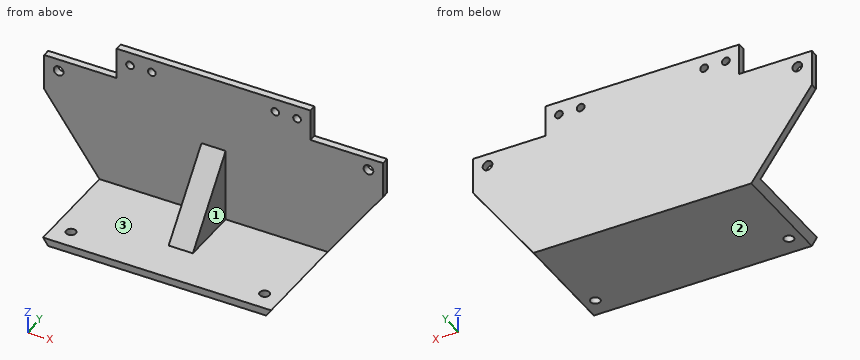
```python
from build123d import *

# Parameters (mm, degrees)
EXTRUDE_1_DEPTH     = 140
CUT_EXTRUDE_1_REACH = 152.354
SKETCH_2_R          = 2
CUT_EXTRUDE_2_REACH = 151.164
SKETCH_3_R          = 2
CUT_EXTRUDE_3_DEPTH = 150.164338902
RIB_2_REACH         = 79.661
SKETCH_9_WALL_W     = 196.169186172
SKETCH_9_WALL_H     = 10
SKETCH_10_W         = 80
SKETCH_10_H         = 3
EXTRUDE_2_DEPTH     = 13
SKETCH_11_R         = 1.6
CUT_EXTRUDE_4_DEPTH = 3


with BuildPart() as part:
    # 草图1 → 凸台-拉伸1 (new body)
    with BuildSketch(Plane(origin=(0, 0, 0), x_dir=(0, 0, -1), z_dir=(1, 0, 0))):
        Polygon((22, 19.5), (22, -22.5), (25, -22.5), (25, 22.5), (-25, 22.5), (-25, 19.5), align=None)
    extrude(amount=EXTRUDE_1_DEPTH)

    # 草图2 → 切除-拉伸1 (cut, up to next)
    with BuildSketch(Plane(origin=(0, 0, -25), x_dir=(-1, 0, 0), z_dir=(0, 0, -1)), mode=Mode.PRIVATE) as cut_extrude_1_sk1:
        with Locations((-110, -14.5)):
            Circle(SKETCH_2_R)
    cut_extrude_1_tool1 = extrude(cut_extrude_1_sk1.sketch, amount=-CUT_EXTRUDE_1_REACH, mode=Mode.PRIVATE) & part.part
    # 草图2 → 切除-拉伸1 (cut, up to next)
    with BuildSketch(Plane(origin=(0, 0, -25), x_dir=(-1, 0, 0), z_dir=(0, 0, -1)), mode=Mode.PRIVATE) as cut_extrude_1_sk2:
        with Locations((-30, -14.5)):
            Circle(SKETCH_2_R)
    cut_extrude_1_tool2 = extrude(cut_extrude_1_sk2.sketch, amount=-CUT_EXTRUDE_1_REACH, mode=Mode.PRIVATE) & part.part
    add(cut_extrude_1_tool1.solids().sort_by_distance((110, -14.5, -25))[0], mode=Mode.SUBTRACT)
    add(cut_extrude_1_tool2.solids().sort_by_distance((30, -14.5, -25))[0], mode=Mode.SUBTRACT)

    # 草图3 → 切除-拉伸2 (cut, up to next)
    with BuildSketch(Plane(origin=(0, 22.5, 0), x_dir=(1, 0, 0), z_dir=(0, 1, 0)), mode=Mode.PRIVATE) as cut_extrude_2_sk1:
        with Locations(Location((6, -20, 0), (0, 0, 270))):
            Circle(SKETCH_3_R)
    cut_extrude_2_tool1 = extrude(cut_extrude_2_sk1.sketch, amount=-CUT_EXTRUDE_2_REACH, mode=Mode.PRIVATE) & part.part
    # 草图3 → 切除-拉伸2 (cut, up to next)
    with BuildSketch(Plane(origin=(0, 22.5, 0), x_dir=(1, 0, 0), z_dir=(0, 1, 0)), mode=Mode.PRIVATE) as cut_extrude_2_sk2:
        with Locations(Location((134, -20, 0), (0, 0, 270))):
            Circle(SKETCH_3_R)
    cut_extrude_2_tool2 = extrude(cut_extrude_2_sk2.sketch, amount=-CUT_EXTRUDE_2_REACH, mode=Mode.PRIVATE) & part.part
    add(cut_extrude_2_tool1.solids().sort_by_distance((6, 22.5, 20))[0], mode=Mode.SUBTRACT)
    add(cut_extrude_2_tool2.solids().sort_by_distance((134, 22.5, 20))[0], mode=Mode.SUBTRACT)

    # 草图4 → 切除-拉伸3 (cut, through all)
    with BuildSketch(Plane(origin=(0, 22.5, 0), x_dir=(1, 0, 0), z_dir=(0, 1, 0))):
        Polygon((140, 25), (115, 25), (140, -10), align=None)
        Polygon((25, 25), (0, 25), (0, -10), align=None)
    extrude(amount=-CUT_EXTRUDE_3_DEPTH, mode=Mode.SUBTRACT)

    # 草图9 wall → 筋2 (add, up to next)
    with BuildSketch(Plane(origin=(70, 7.303048218, -6.883599508), x_dir=(0, 0.627949157595, 0.778254364251), z_dir=(0, 0.778254364251, -0.627949157595)), mode=Mode.PRIVATE) as rib_2_sk1:
        Rectangle(SKETCH_9_WALL_W, SKETCH_9_WALL_H)
    rib_2_tool1 = extrude(rib_2_sk1.sketch, amount=RIB_2_REACH, mode=Mode.PRIVATE) - part.part
    add(rib_2_tool1.solids().sort_by_distance((70, 7.303048218, -6.883599508))[0])

    # 草图10 → 凸台-拉伸2 (add)
    with BuildSketch(Plane.XY.offset(25)):
        with Locations((70, 21)):
            Rectangle(SKETCH_10_W, SKETCH_10_H)
    extrude(amount=EXTRUDE_2_DEPTH)

    # 草图11 → 切除-拉伸4 (cut)
    with BuildSketch(Plane(origin=(0, 22.5, 0), x_dir=(1, 0, 0), z_dir=(0, 1, 0))):
        with Locations(Location((35.5, -32.5, 0), (0, 0, 270))):
            Circle(SKETCH_11_R)
        with Locations(Location((44.5, -32.5, 0), (0, 0, 270))):
            Circle(SKETCH_11_R)
        with Locations(Location((95.5, -32.5, 0), (0, 0, 270))):
            Circle(SKETCH_11_R)
        with Locations(Location((104.5, -32.5, 0), (0, 0, 270))):
            Circle(SKETCH_11_R)
    extrude(amount=-CUT_EXTRUDE_4_DEPTH, mode=Mode.SUBTRACT)


solid = part.part
```
The listing builds one solid part. Answer for the finished solid, in the listing's coordinates (mm). Face numbers are marked on the shaded views. A direction names the side the tool comes from. Round coordinates to 2 decimals unless told otherwise and drop trailing zeros. Loops run counter-clockwise (first coordinate to the right, second up) from the corner with the lowest first, then second, coordinate; pieces in that order, holes last.
Q1. Section C-C, the plane x = 95.5 is taken. Determine the outline of the cut face in (y, z).
Q2. Section A-A, the plane z = 20 is taken. Determine the outline of the cut face in (x, y).
Q3. Find the intervals of material crossed by line 1 (X direction, y = 20.3, z = 32.5); line 2 (Y direction, x = 110, z = -23.85); line 3 (X direction, y = 21, z = 20), in increasing order.
Q4. Section B-B, the plane y = -14.5 is taken. Determine the outline of the cut face in (x, z), then the cut area to 3 significant figures.
Q5. Which of the six approach directions +Z, -Z, +X, -X, +Y, -Y give full straight-line access (tool end or side, diameter ignored) to the marked faces 1, 2 and 3?
Q6. Section D-D, the plane z = 32.5 is taken. Determine the outline of the cut face in (x, y).
Q7. Given pin 1 Ø4 at (x, z) = (94.5, 2.5) entering from -Y; pin 2 Ø7.5 at (y, z) = (1.5, -9) entering from +X; pin 3 Ø3.5 at (y, z) = (21.5, 32) entering from -X; pin 4 Ø3 at (x, z) = (6, 20) entering from +Y, each flat-ended and moving along its own axis, determine where each tip first touches the part or whether it passes through.
Completed:
1. outline: (-22.5, -25) - (22.5, -25) - (22.5, 30.9) - (19.5, 30.9) - (19.5, -22) - (-22.5, -22) - close; (19.5, 34.1) - (22.5, 34.1) - (22.5, 38) - (19.5, 38) - close
2. outline: (0, 19.5) - (4, 19.5) - (4, 22.5) - (0, 22.5) - close; (8, 19.5) - (132, 19.5) - (132, 22.5) - (8, 22.5) - close; (136, 19.5) - (140, 19.5) - (140, 22.5) - (136, 22.5) - close
3. line 1: x = 30 to 33.9, 37.1 to 42.9, 46.1 to 93.9, 97.1 to 102.9, 106.1 to 110
3. line 2: y = -22.5 to -16.5, -12.5 to 22.5
3. line 3: x = 0 to 4, 8 to 132, 136 to 140
4. outline: (22.86, -22) - (25, -25) - (28, -25) - (28, -22) - close; (32, -25) - (108, -25) - (108, -22) - (32, -22) - close; (112, -25) - (115, -25) - (117.14, -22) - (112, -22) - close
4. area: 252 mm2
5. face 1: +Z, +X, -Y
5. face 2: -Z, +X, -X, +Y, -Y
5. face 3: +Z, -Y
6. outline: (30, 19.5) - (33.9, 19.5) - (33.9, 22.5) - (30, 22.5) - close; (37.1, 19.5) - (42.9, 19.5) - (42.9, 22.5) - (37.1, 22.5) - close; (46.1, 19.5) - (93.9, 19.5) - (93.9, 22.5) - (46.1, 22.5) - close; (97.1, 19.5) - (102.9, 19.5) - (102.9, 22.5) - (97.1, 22.5) - close; (106.1, 19.5) - (110, 19.5) - (110, 22.5) - (106.1, 22.5) - close
7. pin 1: stops at y = 19.5
7. pin 2: stops at x = 75
7. pin 3: stops at x = 30
7. pin 4: passes through
